Check sheet for the modelled part. Datum: model origin and axes. Units: mm. A direction names the side the tool comes from. Round coordinates to 2 decimals unless told otherwise and drop trailing zeros. Write each loop counter-clockwise with the first axis right and the second up, starting at its lowest first coordinate (ties: lowest second). Pieces come first, ordered by that corner, then holes. Notation, with made-up numbers: (-13.75, 55) -> (0.25, 55) arc R12 ccw to (0.25, 76) -> close; hole circle Ø8 at (21.5, 62). An arc over 180 degrees is marked (long way). One line per item, written item: value. Start each with the question number.
```python
from build123d import *

# Parameters (mm, degrees)
BOSS_EXTRUDE1_DEPTH = 46.25
FILLET1_R           = 0.5
BOSS_EXTRUDE2_START = 1
BOSS_EXTRUDE2_DEPTH = 1
SKETCH3_R           = 2
CUT_EXTRUDE1_DEPTH  = 21


with BuildPart() as part:
    # Sketch1 → Boss-Extrude1 (new, symmetric)
    with BuildSketch(Plane(origin=(0, 0, 0), x_dir=(0, 1, 0), z_dir=(0, 0, 1))):
        with BuildLine():
            Line((-26.9, 13.95), (-26.4, 13.95))
            Line((-26.4, 13.95), (-26.4, 15.95))
            Line((-26.4, 15.95), (-26.9, 15.95))
            ThreePointArc((-26.9, 15.95), (-31.213351365, 14.163351365), (-33, 9.85))
            Line((-33, 9.85), (-33, -9.85))
            ThreePointArc((-33, -9.85), (-31.213351365, -14.163351365), (-26.9, -15.95))
            Line((-26.9, -15.95), (26.9, -15.95))
            Line((26.9, -15.95), (43, -15.95))
            Line((43, -15.95), (43, -13.95))
            Line((43, -13.95), (35, -13.95))
            ThreePointArc((35, -13.95), (33.585786438, -13.364213562), (33, -11.95))
            Line((33, -11.95), (33, -9.85))
            Line((33, -9.85), (33, 9.85))
            ThreePointArc((33, 9.85), (31.213351365, 14.163351365), (26.9, 15.95))
            Line((26.9, 15.95), (26.4, 15.95))
            Line((26.4, 15.95), (26.4, 13.95))
            Line((26.4, 13.95), (26.9, 13.95))
            ThreePointArc((26.9, 13.95), (29.799137803, 12.749137803), (31, 9.85))
            Line((31, 9.85), (31, -9.85))
            ThreePointArc((31, -9.85), (29.799137803, -12.749137803), (26.9, -13.95))
            Line((26.9, -13.95), (-26.9, -13.95))
            ThreePointArc((-26.9, -13.95), (-29.799137803, -12.749137803), (-31, -9.85))
            Line((-31, -9.85), (-31, 9.85))
            ThreePointArc((-31, 9.85), (-29.799137803, 12.749137803), (-26.9, 13.95))
        make_face()
    extrude(amount=BOSS_EXTRUDE1_DEPTH, both=True)

    # Fillet1
    fillet1_edges = [part.edges().sort_by_distance(p)[0] for p in [
        (-15.95, 26.4, 0),
        (-13.95, 26.4, 0),
        (-13.95, -26.4, 0),
        (-15.95, -26.4, 0),
    ]]
    fillet(fillet1_edges, radius=FILLET1_R - 0.0001)  # a hair under: the kernel refuses the full size

    # Sketch2 → Boss-Extrude2 (add)
    with BuildSketch(Plane.XY.offset(46.25).offset(BOSS_EXTRUDE2_START)):
        with BuildLine():
            Line((-13.371363372, -29), (13.371363372, -29))
            ThreePointArc((13.371363372, -29), (13.80269464, -27.989130427), (13.95, -26.9))
            Line((13.95, -26.9), (13.95, 26.9))
            ThreePointArc((13.95, 26.9), (12.749137803, 29.799137803), (9.85, 31))
            Line((9.85, 31), (-9.85, 31))
            ThreePointArc((-9.85, 31), (-12.749137803, 29.799137803), (-13.95, 26.9))
            ThreePointArc((-13.95, 26.9), (-14.096446609, 26.546446609), (-14.45, 26.4))
            Line((-14.45, 26.4), (-15.45, 26.4))
            ThreePointArc((-15.45, 26.4), (-15.803553391, 26.546446609), (-15.95, 26.9))
            ThreePointArc((-15.95, 26.9), (-14.163351365, 31.213351365), (-9.85, 33))
            Line((-9.85, 33), (11.95, 33))
            ThreePointArc((11.95, 33), (13.364213562, 33.585786438), (13.95, 35))
            Line((13.95, 35), (13.95, 43))
            Line((13.95, 43), (15.95, 43))
            Line((15.95, 43), (15.95, -26.9))
            ThreePointArc((15.95, -26.9), (14.163351365, -31.213351365), (9.85, -33))
            Line((9.85, -33), (-9.85, -33))
            ThreePointArc((-9.85, -33), (-14.163351365, -31.213351365), (-15.95, -26.9))
            ThreePointArc((-15.95, -26.9), (-15.803553391, -26.546446609), (-15.45, -26.4))
            Line((-15.45, -26.4), (-14.45, -26.4))
            ThreePointArc((-14.45, -26.4), (-14.096446609, -26.546446609), (-13.95, -26.9))
            ThreePointArc((-13.95, -26.9), (-13.80269464, -27.989130427), (-13.371363372, -29))
        make_face()
    boss_extrude2 = extrude(amount=-BOSS_EXTRUDE2_DEPTH)

    # Mirror1: Boss-Extrude2 across plane
    add(boss_extrude2.mirror(Plane.XY))

    # Sketch3 → Cut-Extrude1 (cut)
    with BuildSketch(Plane(origin=(13.95, 0, 0), x_dir=(0, -1, 0), z_dir=(-1, 0, 0))):
        with Locations(Location((-39, 32, 0), (0, 0, 90))):
            Circle(SKETCH3_R)
        with Locations(Location((-39, -32, 0), (0, 0, 90))):
            Circle(SKETCH3_R)
    extrude(amount=-CUT_EXTRUDE1_DEPTH, mode=Mode.SUBTRACT)


solid = part.part
```
1. Cross-section at C-C (x = 4). Record the cut outline in (y, z), plus the area to 3 significant figures.
2. Release check for a two-part mould opening along Y. For faces 4 (the face through (15, 43, -1)), 5 (the face through (0, -31, 1)), 6 (the face through (14.211, -31.166, -0.662)), 7 (the face through (15.95, 9, -1)) record: +Y half, -Y half, draft (parallel to the pull), parting line (faces both ways), or undercut.
3. Material ranges on probe 1 along Y at (x, z) = (-1, -8); probe 2 along X at (y, z) = (-0.5, -39.5), recorded low to high.
4. Depth check by flat-ended pin: pin 1 Ø10 at (y, z) = (35, -0.5) entering from -X; pin 2 Ø0.8 at (x, z) = (-14.5, 4.5) entering from +Y; pin 3 Ø1.1 at (x, z) = (-15, -16) entering from -Y; pin 4 Ø12 at (x, y) = (7, -20.5) entering from -Z. Enter the tip coordinate at first touch or a pass-through.
5. Cross-section at D-D (y = -20). Record the cut outline in (x, z).
6. Cross-section at A-A (y = 39). Record the cut outline in (x, z), plus the area to 3 significant figures.
7. Access from +Z, -Z, +X, -X, +Y, -Y to the whole of each face (thin tool, end or side, straight path). Record for faces 1 (the face through (0, -30, -46.25)), 2 (the face through (1, 33, -1)), 3 (the face through (0, 31, -1)).
Working result:
1. outline: (-33, -47.25) -> (-29, -47.25) -> (-29, -46.25) -> (-31, -46.25) -> (-31, 46.25) -> (-29, 46.25) -> (-29, 47.25) -> (-33, 47.25) -> close; (31, -47.25) -> (33, -47.25) -> (33, 47.25) -> (31, 47.25) -> close
1. area: 382 mm^2
2. face 4: +Y half
2. face 5: undercut
2. face 6: -Y half
2. face 7: draft
3. probe 1: y = -33 to -31, 31 to 33
3. probe 2: x = 13.95 to 15.95
4. pin 1: stops at x = -15.1
4. pin 2: stops at y = 31.28
4. pin 3: stops at y = -30.91
4. pin 4: passes through
5. outline: (13.95, -47.25) -> (15.95, -47.25) -> (15.95, 47.25) -> (13.95, 47.25) -> close
6. outline: (13.95, -47.25) -> (15.95, -47.25) -> (15.95, -34) -> (13.95, -34) -> close; (13.95, -30) -> (15.95, -30) -> (15.95, 30) -> (13.95, 30) -> close; (13.95, 34) -> (15.95, 34) -> (15.95, 47.25) -> (13.95, 47.25) -> close
6. area: 173 mm^2
7. face 1: none
7. face 2: +Z, -Z, -X, +Y
7. face 3: +Z, -Z
